```python
from build123d import *

# Parameters (mm, degrees)
F0_W     = 76.2
F0_H     = 76.2
F1_DEPTH = 38.1
F3_DEPTH = 76.2
F5_DEPTH = 76.2


with BuildPart() as f1:
    # F0 (on Right) → F1 (new body, symmetric)
    with BuildSketch(Plane.YZ):
        Rectangle(F0_W, F0_H)
    extrude(amount=F1_DEPTH, both=True)

    # F2 (on face) → F3 (cut)
    with BuildSketch(Plane.YZ.offset(38.1)):
        Polygon((38.1, 38.1), (-38.1, 38.1), (-38.1, -38.1), align=None)
    extrude(amount=-F3_DEPTH, mode=Mode.SUBTRACT)

    # F4 (on face) → F5 (cut)
    with BuildSketch(Plane(origin=(0, 0, -38.1), x_dir=(1, 0, 0), z_dir=(0, 0, -1))):
        Polygon((-38.1, -38.1), (38.1, 38.1), (-38.1, 38.1), align=None)
    extrude(amount=-F5_DEPTH, mode=Mode.SUBTRACT)


solid = f1.part
```
Can you work these out from the model? Positions are in its coordinate system, mm. Round coordinates to 2 decimals unless told otherwise and drop trailing zeros. Loops run counter-clockwise (first coordinate to the right, second up) from the corner with the lowest first, then second, coordinate; pieces in that order, holes last.
Item 1: Please list where these lines run through material, in increasing order: L1, parallel to Y at x = -25, z = 8; L2, parallel to Y at x = -26, z = 23; L3, parallel to Z at x = 21.5, y = 7.5.
Item 2: Will these pins go through, and if not, where does the flat tip stop? pin 1 Ø1.5 at (x, z) = (-14, 21) entering from -Y; pin 2 Ø4 at (x, y) = (-9.5, 11.5) entering from +Z; pin 3 Ø1.5 at (x, z) = (1, 16.5) entering from -Y.
Item 3: Suppose I cut it at A-A, the plane x = 29.5. Write out the boundary of the cut face in (y, z).
Item 4: Suppose I cut it at B-B, the plane y = 4. Write out the boundary of the cut face in (x, z).
Reported:
1. L1: y = 25 to 38.1
1. L2: y = 26 to 38.1
1. L3: z = -38.1 to 7.5
2. pin 1: stops at y = 20.25
2. pin 2: stops at z = 13.5
2. pin 3: stops at y = 15.75
3. outline: (-29.5, -38.1) - (38.1, -38.1) - (38.1, 38.1) - (-29.5, -29.5) - close
4. outline: (-4, -38.1) - (38.1, -38.1) - (38.1, 4) - (-4, 4) - close
